Design review of the part built by this model. Coordinates are the model's own, in mm. A direction names the side the tool comes from. Coordinates: 2 decimals unless noted, no trailing zeros. Loops run counter-clockwise (first coordinate to the right, second up) from the corner with the lowest first, then second, coordinate; pieces in that order, holes last. Notation, with made-up numbers: (81, -10) -> (108, -10) arc R32 cw to (108, 24) -> close; hole circle Ø2 at (-28, 8.25). An arc over 180 degrees is marked (long way). Answer as a JSON object with one key per item and string values.
```python
from build123d import *

# Parameters (mm, degrees)
BOSS_EXTRUDE1_DEPTH = 80
SKETCH2_R           = 7.5
CUT_EXTRUDE2_DEPTH  = 632.189353522
SKETCH4_W           = 50
SKETCH4_H           = 260
CUT_EXTRUDE3_DEPTH  = 632.189353668


with BuildPart() as part:
    # Sketch1 → Boss-Extrude1 (new body)
    with BuildSketch(Plane.XY):
        with BuildLine():
            Line((-280, 0), (-280, -20))
            Line((-280, -20), (-270, -20))
            Line((-270, -20), (-270, 0))
            ThreePointArc((-270, 0), (0, 270), (270, 0))
            Line((270, 0), (270, -20))
            Line((270, -20), (280, -20))
            Line((280, -20), (280, 0))
            ThreePointArc((280, 0), (0, 280), (-280, 0))
        make_face()
    extrude(amount=BOSS_EXTRUDE1_DEPTH)

    # Sketch2 → Cut-Extrude2 (cut, through all)
    with BuildSketch(Plane(origin=(280, 0, 0), x_dir=(0, 0, -1), z_dir=(1, 0, 0))):
        with Locations((-40, 0)):
            Circle(SKETCH2_R)
    extrude(amount=-CUT_EXTRUDE2_DEPTH, mode=Mode.SUBTRACT)

    # Sketch4 → Cut-Extrude3 (cut, through all)
    with BuildSketch(Plane(origin=(280, 0, 0), x_dir=(0, 0, -1), z_dir=(1, 0, 0))):
        with Locations((-40, 150)):
            Rectangle(SKETCH4_W, SKETCH4_H)
    extrude(amount=-CUT_EXTRUDE3_DEPTH, mode=Mode.SUBTRACT)


solid = part.part
```
1) Wall thickness on probe 1 along Z at (x, y) = (272, 0); probe 2 along Y at (x, z) = (277, 40); probe 3 along X at (y, z) = (236.5, 4.5): over which ranges is each line inside the solid? List them lowest first.
Completed:
{"probe 1": "0 to 32.5, 47.5 to 80", "probe 2": "-20 to -7.5, 7.5 to 20", "probe 3": "-149.89 to -130.26, 130.26 to 149.89"}
2) The part is to be moulded in two halves that separate along Z. For faces 1 (the flat face through (-1, 275, 80)), 2 (the flat face through (270, -10, 39)), 3 (the flat face through (1, 275, 15)), 4 (the flat face through (-274, 20, 40)), say which applies: pulls with the +Z half, pulls with the -Z half, needs draft (parallel to the pull), parting line crosses it, or undercut.
Completed:
{"face 1": "pulls with the +Z half", "face 2": "needs draft", "face 3": "undercut", "face 4": "undercut"}
3) Add section D-D, the plane x = 184.5. Give the boundary of the cut face in (y, z).
Completed:
{"outline": "(197.13, 0) -> (210.62, 0) -> (210.62, 15) -> (197.13, 15) -> close; (197.13, 65) -> (210.62, 65) -> (210.62, 80) -> (197.13, 80) -> close"}
4) Add section B-B, the plane z = 24. Give the boundary of the cut face in (x, y), and give its area (3 significant figures).
Completed:
{"outline": "(-280, -20) -> (-270, -20) -> (-270, 0) arc R270 cw to (-269.26, 20) -> (-279.28, 20) arc R280 ccw to (-280, 0) -> close; (269.26, 20) arc R270 cw to (270, 0) -> (270, -20) -> (280, -20) -> (280, 0) arc R280 ccw to (279.28, 20) -> close", "area": "800 mm²"}
5) Clearance check with flat-ended pins moving along their axes: pin 1 Ø3 at (x, z) = (274.5, 30) entering from +Y; pin 2 Ø13.5 at (y, z) = (0, 40) entering from -X. State where each tip first meets the part, or that it passes through.
Completed:
{"pin 1": "y = 20", "pin 2": "through"}
6) Add section A-A, the plane x = 0. Give the boundary of the cut face in (y, z), and give its area (3 significant figures).
Completed:
{"outline": "(270, 0) -> (280, 0) -> (280, 15) -> (270, 15) -> close; (270, 65) -> (280, 65) -> (280, 80) -> (270, 80) -> close", "area": "300 mm²"}
7) For faces 5 (the flat face through (275, -20, 39)), 6 (the flat face through (1, 275, 65)), 7 (the flat face through (-270, -10, 39)), list the 3-axis set-ups (+Z, -Z, +X, -X, +Y, -Y) from which the entire face can be reached by the end or side of a thin tool; tool diameter is ignored.
Completed:
{"face 5": "+Z, -Z, +X, -X, -Y", "face 6": "+X, -X, +Y", "face 7": "+Z, -Z, -Y"}
8) Add section C-C, the plane y = 114.5. Give the boundary of the cut face in (x, z).
Completed:
{"outline": "(-255.52, 0) -> (-244.52, 0) -> (-244.52, 15) -> (-255.52, 15) -> close; (-255.52, 65) -> (-244.52, 65) -> (-244.52, 80) -> (-255.52, 80) -> close; (244.52, 0) -> (255.52, 0) -> (255.52, 15) -> (244.52, 15) -> close; (244.52, 65) -> (255.52, 65) -> (255.52, 80) -> (244.52, 80) -> close"}
